```python
from build123d import *

# Parameters (mm, degrees)
SKETCH_1_R          = 1.6
EXTRUDE_1_DEPTH     = 1
SKETCH_2_R          = 1
CUT_EXTRUDE_1_DEPTH = 10
FILLET_1_R          = 1
SKETCH_3_W          = 0.5
SKETCH_3_H          = 12.9
SKETCH_3_H_2        = 60
CUT_EXTRUDE_2_DEPTH = 154.412548379
FILLET_2_R          = 0.5


with BuildPart() as part:
    # 草图1 → 凸台-拉伸1 (new body)
    with BuildSketch(Plane.XY):
        Polygon((0, 0), (0, 12.9), (146, 12.9), (146, -47.1), (67.7, -47.1), (67.7, 0), align=None)
        with Locations(Location((47.25, 3, 0), (0, 0, 180))):
            Circle(SKETCH_1_R, mode=Mode.SUBTRACT)
        with Locations(Location((27.25, 3, 0), (0, 0, 180))):
            Circle(SKETCH_1_R, mode=Mode.SUBTRACT)
    extrude(amount=EXTRUDE_1_DEPTH)

    # 草图2 → 切除-拉伸1 (cut)
    with BuildSketch(Plane.XY.offset(1)):
        with Locations((67.7, -1)):
            Circle(SKETCH_2_R)
    extrude(amount=-CUT_EXTRUDE_1_DEPTH, mode=Mode.SUBTRACT)

    # 圆角1
    fillet_1_edges = [part.edges().sort_by_distance(p)[0] for p in [
        (67.7, -2, 0.5),
    ]]
    fillet(fillet_1_edges, radius=FILLET_1_R)

    # 草图3 → 切除-拉伸2 (cut, through all)
    with BuildSketch(Plane.XY.offset(1)):
        with Locations((0.25, 6.45)):
            Rectangle(SKETCH_3_W, SKETCH_3_H)
        with Locations((145.75, -17.1)):
            Rectangle(SKETCH_3_W, SKETCH_3_H_2)
    extrude(amount=-CUT_EXTRUDE_2_DEPTH, mode=Mode.SUBTRACT)

    # 圆角2
    fillet_2_edges = [part.edges().sort_by_distance(p)[0] for p in [
        (0.5, 12.9, 0.5),
        (145.5, 12.9, 0.5),
    ]]
    fillet(fillet_2_edges, radius=FILLET_2_R)


solid = part.part
```
Here's how the part is built. I have some questions about the finished solid (model axes, mm). Round coordinates to 2 decimals unless told otherwise and drop trailing zeros. Order: outer loops, then holes, each group sorted by start corner. A loop starts at its lowest first (then second) coordinate and runs counter-clockwise, first axis right, second up. Notation, with made-up numbers: (-12.75, -24) -> (31.25, -24) arc R18 cw to (31.25, -16) -> close; hole circle Ø3 at (14.25, 9). An arc over 180 degrees is marked (long way). Use a Markdown table: item, result. Add a question column.
(1) For pin 1 Ø2.5 at (x, y) = (47.25, 3) entering from +Z; pin 2 Ø0.5 at (y, z) = (-20.5, 0.5) entering from -X; pin 3 Ø4 at (x, y) = (27.25, 3) entering from +Z, each with a flat end and sliding along its axis, tell me the tip position at first contact or that it passes through.
(2) Suppose I cut it at A-A, the plane x = 47.25. Please give me the cut outline in (y, z).
(3) Suppose I cut it at D-D, the plane x = 17. Please give me the cut outline in (y, z).
(4) Suppose I cut it at B-B, the plane z = 0.85. Please give me the cut outline in (x, y).
(5) Suppose I cut it at C-C, the plane y = 3. Please give me the cut outline in (x, z), and give its area (3 significant figures).
(6) I need wall thicknesses on line 1 along Y through (x, z) = (27.25, 0.6); line 2 along X through (y, z) = (3, 0.75); line 3 along X through (y, z) = (2, 0.15). Which ranges of each line are inside material? Lowest first, please.
(7) If we mould it in two halves opening along Y, with no side actions, what happens to faces 1 (the face through (90, -10, 0)), 2 (the face through (28.43, 1.92, 0.49))? For each: released by +Y, released by -Y, zero draft, split by the parting line, or undercut.
Verdict:
| question | item | result |
|---|---|---|
| 1 | pin 1 | through |
| 1 | pin 2 | x = 67.7 |
| 1 | pin 3 | z = 1 |
| 2 | outline | (0, 0) -> (1.4, 0) -> (1.4, 1) -> (0, 1) -> close; (4.6, 0) -> (12.9, 0) -> (12.9, 1) -> (4.6, 1) -> close |
| 3 | outline | (0, 0) -> (12.9, 0) -> (12.9, 1) -> (0, 1) -> close |
| 4 | outline | (0.5, 0) -> (67.7, 0) arc R1 cw to (68.2, -1.87) arc R1 ccw to (67.7, -2.73) -> (67.7, -47.1) -> (145.5, -47.1) -> (145.5, 12.4) arc R0.5 ccw to (145, 12.9) -> (1, 12.9) arc R0.5 ccw to (0.5, 12.4) -> close; hole circle Ø3.2 at (27.25, 3); hole circle Ø3.2 at (47.25, 3) |
| 5 | outline | (0.5, 0) -> (25.65, 0) -> (25.65, 1) -> (0.5, 1) -> close; (28.85, 0) -> (45.65, 0) -> (45.65, 1) -> (28.85, 1) -> close; (48.85, 0) -> (145.5, 0) -> (145.5, 1) -> (48.85, 1) -> close |
| 5 | area | 139 mm2 |
| 6 | line 1 | 0 to 1.4, 4.6 to 12.9 |
| 6 | line 2 | 0.5 to 25.65, 28.85 to 45.65, 48.85 to 145.5 |
| 6 | line 3 | 0.5 to 26, 28.5 to 46, 48.5 to 145.5 |
| 7 | face 1 | zero draft |
| 7 | face 2 | undercut |
